```python
from build123d import *

# Parameters (mm, degrees)
SKETCH_1_R               = 93.03002178900209
EXTRUDE_1_DEPTH          = 4
SKETCH_2_R               = 2.4
EXTRUDE_2_DEPTH          = 45
SKETCH_3_R               = 5
EXTRUDE_3_DEPTH          = 5
SKETCH_4_R               = 2.3999999999999937
EXTRUDE_4_DEPTH          = 12.999999999999998
SKETCH_5_R               = 4.9999999999999964
EXTRUDE_5_DEPTH          = 4.999999999999997
SKETCH_6_R               = 2.3999999999999932
EXTRUDE_6_DEPTH          = 20.200000000000017
SKETCH_7_R               = 4.9999999999999964
EXTRUDE_7_DEPTH          = 14
CUT_EXTRUDE_1_REACH      = 141.047
SKETCH_8_R               = 5.153202095824808
SKETCH_9_R               = 2.5515156643505628
SKETCH_9_R_2             = 2.551515664350585
SKETCH_9_R_3             = 2.551515664350554
SKETCH_9_R_4             = 2.5515156643508896
CUT_EXTRUDE_3_DEPTH      = 5.9999999999999964
CUT_EXTRUDE_4_REACH      = 141.024
PATTERN_CIRCULAR_1_COUNT = 6
FILLET_1_R               = 5


with BuildPart() as part:
    # 草图1 → 凸台-拉伸1 (new body)
    with BuildSketch(Plane(origin=(0, 0, 0), x_dir=(0, 0, -1), z_dir=(1, 0, 0))):
        Circle(SKETCH_1_R)
    extrude(amount=EXTRUDE_1_DEPTH)

    # 草图2 → 凸台-拉伸2 (add)
    with BuildSketch(Plane(origin=(4, 0, 0), x_dir=(0, 0, -1), z_dir=(1, 0, 0))):
        with Locations(Location((0, 0, 0), (0, 0, 180))):
            Circle(SKETCH_2_R)
    extrude(amount=EXTRUDE_2_DEPTH)

    # 草图3 → 凸台-拉伸3 (add)
    with BuildSketch(Plane(origin=(4, 0, 0), x_dir=(0, 0, -1), z_dir=(1, 0, 0))):
        Circle(SKETCH_3_R)
    extrude(amount=EXTRUDE_3_DEPTH)

    # 草图4 → 凸台-拉伸4 (add)
    with BuildSketch(Plane(origin=(4, 0, 0), x_dir=(0, 0, -1), z_dir=(1, 0, 0))):
        with Locations((62.35382907247964, -35.9999999999998)):
            Circle(SKETCH_4_R)
    extrude(amount=EXTRUDE_4_DEPTH)

    # 草图5 → 凸台-拉伸5 (add)
    with BuildSketch(Plane(origin=(4, 0, 0), x_dir=(0, 0, -1), z_dir=(1, 0, 0))):
        with Locations((62.35382907247964, -35.9999999999998)):
            Circle(SKETCH_5_R)
    extrude(amount=EXTRUDE_5_DEPTH)

    # 草图6 → 凸台-拉伸6 (add)
    with BuildSketch(Plane(origin=(4, 0, 0), x_dir=(0, 0, -1), z_dir=(1, 0, 0))):
        with Locations((-62.35382907247939, -36.00000000000031)):
            Circle(SKETCH_6_R)
    extrude(amount=EXTRUDE_6_DEPTH)

    # 草图7 → 凸台-拉伸7 (add)
    with BuildSketch(Plane(origin=(4, 0, 0), x_dir=(0, 0, -1), z_dir=(1, 0, 0))):
        with Locations((-62.35382907247939, -36.00000000000031)):
            Circle(SKETCH_7_R)
    extrude(amount=EXTRUDE_7_DEPTH)

    # 草图8 → 切除-拉伸1 (cut, up to next)
    with BuildSketch(Plane(origin=(4, 0, 0), x_dir=(0, 0, -1), z_dir=(1, 0, 0)), mode=Mode.PRIVATE) as cut_extrude_1_sk1:
        with Locations((0, 93.03002178900209)):
            Circle(SKETCH_8_R)
    cut_extrude_1_tool1 = extrude(cut_extrude_1_sk1.sketch, amount=-CUT_EXTRUDE_1_REACH, mode=Mode.PRIVATE) & part.part
    add(cut_extrude_1_tool1.solids().sort_by_distance((4, 93.030022, 0))[0], mode=Mode.SUBTRACT)

    # 草图9 → 切除-拉伸3 (cut)
    with BuildSketch(Plane(origin=(4, 0, 0), x_dir=(0, 0, -1), z_dir=(1, 0, 0))):
        with Locations((3.47e-15, 93.03002178900209)):
            Circle(SKETCH_9_R)
        with Locations((80.56636218389566, 46.515010894501074)):
            Circle(SKETCH_9_R_2)
        with Locations((80.56636218389568, -46.51501089450103)):
            Circle(SKETCH_9_R_3)
        with Locations((8.67e-15, -93.03002178900209)):
            Circle(SKETCH_9_R)
        with Locations((-80.56636218389565, -46.51501089450109)):
            Circle(SKETCH_9_R_3)
        with Locations((-80.56636218389569, 46.51501089450098)):
            Circle(SKETCH_9_R_4)
    extrude(amount=-CUT_EXTRUDE_3_DEPTH, mode=Mode.SUBTRACT)

    # 草图10 → 切除-拉伸4 (cut, up to next)
    with BuildSketch(Plane(origin=(4, 0, 0), x_dir=(0, 0, -1), z_dir=(1, 0, 0)), mode=Mode.PRIVATE) as cut_extrude_4_sk1:
        with BuildLine():
            Line((-10.407514658464736, 18.02634416897966), (-10.407514658464395, 76.04625246317465))
            ThreePointArc((-10.407514658464395, 76.04625246317465), (-38.37756139679427, 66.47188620984315), (-60.65422916648111, 47.03629831607756))
            Line((-60.65422916648111, 47.03629831607756), (-10.407514658464736, 18.02634416897966))
        make_face()
    cut_extrude_4_tool1 = extrude(cut_extrude_4_sk1.sketch, amount=-CUT_EXTRUDE_4_REACH, mode=Mode.PRIVATE) & part.part
    cut_extrude_4 = cut_extrude_4_tool1.solids().sort_by_distance((4, 49.214145, 28.4138))[0]
    add(cut_extrude_4, mode=Mode.SUBTRACT)

    # 阵列(圆周)1: 切除-拉伸4 ×6 about axis
    pattern_circular_1_axis = Axis((0, -1e-16, -8.9e-16), (1, 0, 0))
    for i in range(1, PATTERN_CIRCULAR_1_COUNT):
        add(cut_extrude_4.rotate(pattern_circular_1_axis, i * 360 / PATTERN_CIRCULAR_1_COUNT), mode=Mode.SUBTRACT)

    # 圆角1
    fillet_1_edges = [part.edges().sort_by_distance(p)[0] for p in [
        (2, 18.02634416897966, 10.407514658464736),
        (2, 47.03629831607757, 60.65422916648111),
        (2, 76.04625246317465, 10.407514658464397),
        (2, -18.026344168979215, 10.407514658465503),
        (2, -76.04625246317445, 10.407514658465852),
        (2, -47.036298316076405, 60.654229166482004),
        (2, 4.4326e-13, 20.815029316930236),
        (2, -29.009954147096884, 71.06174382494694),
        (2, 29.00995414709824, 71.06174382494639),
        (2, -4.5413e-13, -20.815029316930236),
        (2, 29.009954147096852, -71.06174382494696),
        (2, -29.00995414709827, -71.06174382494638),
        (2, -18.02634416897966, -10.407514658464736),
        (2, -47.03629831607758, -60.6542291664811),
        (2, -76.04625246317465, -10.40751465846439),
        (2, 18.026344168979218, -10.4075146584655),
        (2, 76.04625246317445, -10.407514658465825),
        (2, 47.036298316076426, -60.65422916648199),
    ]]
    fillet(fillet_1_edges, radius=FILLET_1_R)


solid = part.part
```
Could you check a few things on this model? Use its own coordinates, in mm. A direction names the side the tool comes from. Coordinates: 2 decimals unless noted, no trailing zeros. Write each loop counter-clockwise with the first axis right and the second up, starting at its lowest first coordinate (ties: lowest second). Pieces come first, ordered by that corner, then holes. Notation, with made-up numbers: (-13.5, 55.5) -> (44.5, 55.5) arc R17 ccw to (44.5, 66.5) -> close; hole circle Ø3 at (39, 67.25). An arc over 180 degrees is marked (long way). Return JSON: item names as keys, results as strings.
(1) I need wall thicknesses on L1, parallel to X at y = -15, z = -78. Which ranges of the line are inside material? Lowest first, please.
Numbers:
{"L1": "x = 0 to 4"}
(2) Imagine slicing it at A-A, the plane y = 0. Please give me the cut outline in (x, z), then the cut area to 3 significant figures.
Numbers:
{"outline": "(0, -93.03) -> (4, -93.03) -> (4, -76.76) -> (0, -76.76) -> close; (0, -25.82) -> (4, -25.82) -> (4, -5) -> (9, -5) -> (9, -2.4) -> (49, -2.4) -> (49, 2.4) -> (9, 2.4) -> (9, 5) -> (4, 5) -> (4, 25.82) -> (0, 25.82) -> close; (0, 76.76) -> (4, 76.76) -> (4, 93.03) -> (0, 93.03) -> close", "area": "579 mm2"}
(3) Imagine slicing it at C-C, the plane x = 21. Please give me the cut outline in (y, z).
Numbers:
{"outline": "circle Ø4.8 at (-36, 62.35); circle Ø4.8 at (0, 0)"}
(4) I'm going to push flat-ended pins straight in: pin 1 (1.5 mm diameter, centred on y = 41, z = -10, fed in from +X); pin 2 (5 mm diameter, centred on y = -36.5, z = 60.5, fed in from +X); pin 3 (3 mm diameter, centred on x = 2.5, y = -50, fed in from -Z); pin 4 (11 mm diameter, centred on y = 1, z = 2.5, fed in from +X). Where does each tip first touch, or does it pass through?
Numbers:
{"pin 1": "stops at x = 4", "pin 2": "stops at x = 24.2", "pin 3": "stops at z = -79.26", "pin 4": "stops at x = 49"}
(5) We'd pull the mould along Y, two halves only. Please class faces 1 (the cylindrical face through (1.97, 73.94, 12.23)), 2 (the cylindrical face through (6.46, -4.88, 1.08)), 3 (the flat face through (24.2, -36, 62)): +Y half, -Y half, draft (parallel to the pull), parting line (faces both ways), or undercut.
Numbers:
{"face 1": "undercut", "face 2": "parting line", "face 3": "draft"}
(6) Imagine slicing it at B-B, the plane z = -31.5. Please give me the cut outline in (x, y), then the cut area to 3 significant figures.
Numbers:
{"outline": "(0, -87.53) -> (4, -87.53) -> (4, -69.99) -> (0, -69.99) -> close; (0, -30.2) -> (4, -30.2) -> (4, -6.17) -> (0, -6.17) -> close; (0, 6.17) -> (4, 6.17) -> (4, 30.2) -> (0, 30.2) -> close; (0, 69.99) -> (4, 69.99) -> (4, 87.53) -> (0, 87.53) -> close", "area": "333 mm2"}
(7) Imagine slicing it at D-D, the plane z = 0. Please give me the cut outline in (x, y), then the cut area to 3 significant figures.
Numbers:
{"outline": "(0, -90.48) -> (4, -90.48) -> (4, -5) -> (9, -5) -> (9, -2.4) -> (49, -2.4) -> (49, 2.4) -> (9, 2.4) -> (9, 5) -> (4, 5) -> (4, 87.88) -> (0, 87.88) -> close", "area": "955 mm2"}
(8) Which directions (+Z, -Z, +X, -X, +Y, -Y) give clear straight access to the entire face, cutting with the end or side of a thin tool? Please do faces 4 (the cylindrical face through (12.944, -35.894, -59.956)), 5 (the cylindrical face through (1.972, 22.394, 12.844)), 6 (the cylindrical face through (1.972, 80.228, 47.097)).
Numbers:
{"face 4": "+X", "face 5": "+X, -X", "face 6": "+Z, +X, -X, +Y"}
